```python
from build123d import *

# Parameters (mm, degrees)
ESTRUSIONE_SOTTILE1_DEPTH    = 6
RACCORDO3_R                  = 6
SCHIZZO4_R                   = 2
TAGLIO_ESTRUSIONE1_DEPTH     = 0.75
RACCORDO1_R                  = 0.75
RACCORDO2_R                  = 0.5
TAGLIO_ESTRUSIONE2_DEPTH     = 0.75
SCHIZZO6_R                   = 2
ESTRUSIONE_ESTRUSIONE1_DEPTH = 0.75
ESTRUSIONE_ESTRUSIONE3_DEPTH = 6
RACCORDO3_OF_SPECCHIA2_R     = 6
RACCORDO1_OF_SPECCHIA2_R     = 0.75
RACCORDO2_OF_SPECCHIA2_R     = 0.5
SCHIZZO8_R                   = 2
TAGLIO_ESTRUSIONE3_DEPTH     = 0.75
SCHIZZO9_R                   = 2
TAGLIO_ESTRUSIONE4_DEPTH     = 19


with BuildPart() as part:
    # Schizzo1 → Estrusione-Sottile1 (new, symmetric)
    with BuildSketch(Plane.XY):
        Polygon((0, 13), (0, 0), (-11, 0), (-11, 0.75), (-0.75, 0.75), (-0.75, 13), align=None)
    estrusione_sottile1 = extrude(amount=ESTRUSIONE_SOTTILE1_DEPTH, both=True)

    # Raccordo3
    raccordo3_edges = [part.edges().sort_by_distance(p)[0] for p in [
        (-11, 0.375, 6),
        (-11, 0.375, -6),
        (-0.375, 13, -6),
        (-0.375, 13, 6),
    ]]
    fillet(raccordo3_edges, radius=RACCORDO3_R - 0.0001)  # a hair under: the kernel refuses the full size

    # Schizzo4 → Taglio-Estrusione1 (cut)
    with BuildSketch(Plane(origin=(0, 0.75, 0), x_dir=(1, 0, 0), z_dir=(0, 1, 0))):
        with Locations(Location((-7, 0, 0), (0, 0, 180))):
            Circle(SCHIZZO4_R)
    taglio_estrusione1 = extrude(amount=-TAGLIO_ESTRUSIONE1_DEPTH, mode=Mode.SUBTRACT)

    # Raccordo1
    raccordo1_edges = [part.edges().sort_by_distance(p)[0] for p in [
        (0, 0, 0),
    ]]
    fillet(raccordo1_edges, radius=RACCORDO1_R)

    # Raccordo2
    raccordo2_edges = [part.edges().sort_by_distance(p)[0] for p in [
        (-0.75, 0.75, 0),
    ]]
    fillet(raccordo2_edges, radius=RACCORDO2_R)

    # Schizzo5 → Taglio-Estrusione2 (cut)
    with BuildSketch(Plane.ZY.offset(0.75)):
        with BuildLine():
            Line((2, 9), (2, 3.5))
            ThreePointArc((2, 3.5), (0, 1.5), (-2, 3.5))
            Line((-2, 3.5), (-2, 9))
            ThreePointArc((-2, 9), (0, 11), (2, 9))
        make_face()
    extrude(amount=-TAGLIO_ESTRUSIONE2_DEPTH, mode=Mode.SUBTRACT)

    # Schizzo6 → Estrusione-Estrusione1 (add)
    with BuildSketch(Plane(origin=(0, 0.75, 0), x_dir=(1, 0, 0), z_dir=(0, 1, 0))):
        with BuildLine():
            Line((-4.125, -6), (-7, -6))
            ThreePointArc((-7, -6), (-13, 0), (-7, 6))
            Line((-7, 6), (-4.125, 6))
            Line((-4.125, 6), (-4.125, -6))
        make_face()
        with Locations(Location((-7, 0, 0), (0, 0, 180))):
            Circle(SCHIZZO6_R, mode=Mode.SUBTRACT)
    estrusione_estrusione1 = extrude(amount=-ESTRUSIONE_ESTRUSIONE1_DEPTH)

    # Schizzo7 → Estrusione-Estrusione3 (add, symmetric)
    with BuildSketch(Plane.XY):
        with BuildLine():
            Line((-0.75, 13), (-0.75, 7))
            Line((-0.75, 7), (-0.75, 1.25))
            ThreePointArc((-0.75, 1.25), (-0.896446609, 0.896446609), (-1.25, 0.75))
            Line((-1.25, 0.75), (-4.125, 0.75))
            Line((-4.125, 0.75), (-4.125, 0))
            Line((-4.125, 0), (-0.75, 0))
            ThreePointArc((-0.75, 0), (-0.219669914, 0.219669914), (0, 0.75))
            Line((0, 0.75), (0, 7))
            Line((0, 7), (0, 13))
            Line((0, 13), (0, 13.5))
            ThreePointArc((0, 13.5), (0.073223305, 13.676776695), (0.25, 13.75))
            Line((0.25, 13.75), (5.5, 13.75))
            Line((5.5, 13.75), (5.5, 14.5))
            Line((5.5, 14.5), (0.25, 14.5))
            ThreePointArc((0.25, 14.5), (-0.457106781, 14.207106781), (-0.75, 13.5))
            Line((-0.75, 13.5), (-0.75, 13))
        make_face()
    estrusione_estrusione3 = extrude(amount=ESTRUSIONE_ESTRUSIONE3_DEPTH, both=True)


with BuildPart() as specchia2_1:
    # Specchia2: Estrusione-Sottile1 across plane
    add(estrusione_sottile1.mirror(Plane(origin=(5.5, 14.5, 6), x_dir=(0, 0, 1), z_dir=(-1, 0, 0))))

    # Specchia2 2: Taglio-Estrusione1 across plane
    add(taglio_estrusione1.mirror(Plane(origin=(5.5, 14.5, 6), x_dir=(0, 0, 1), z_dir=(-1, 0, 0))), mode=Mode.SUBTRACT)

    # Raccordo3 of Specchia2
    raccordo3_of_specchia2_edges = [specchia2_1.edges().sort_by_distance(p)[0] for p in [
        (22, 0.375, 6),
        (22, 0.375, -6),
        (11.375, 13, -6),
        (11.375, 13, 6),
    ]]
    fillet(raccordo3_of_specchia2_edges, radius=RACCORDO3_OF_SPECCHIA2_R - 0.0001)  # a hair under: the kernel refuses the full size

    # Raccordo1 of Specchia2
    raccordo1_of_specchia2_edges = [specchia2_1.edges().sort_by_distance(p)[0] for p in [
        (11, 0, 0),
    ]]
    fillet(raccordo1_of_specchia2_edges, radius=RACCORDO1_OF_SPECCHIA2_R)

    # Raccordo2 of Specchia2
    raccordo2_of_specchia2_edges = [specchia2_1.edges().sort_by_distance(p)[0] for p in [
        (11.75, 0.75, 0),
    ]]
    fillet(raccordo2_of_specchia2_edges, radius=RACCORDO2_OF_SPECCHIA2_R)


with BuildPart() as specchia2_3_1:
    # Specchia2 3: Estrusione-Estrusione1, Estrusione-Estrusione3 across plane
    add(estrusione_estrusione1.mirror(Plane(origin=(5.5, 14.5, 6), x_dir=(0, 0, 1), z_dir=(-1, 0, 0))))
    add(estrusione_estrusione3.mirror(Plane(origin=(5.5, 14.5, 6), x_dir=(0, 0, 1), z_dir=(-1, 0, 0))))


with BuildPart() as part_1:
    add(part.part)

    # Specchia2 united with what the copies to: union Specchia2_1, Specchia2 3_1
    add(specchia2_1.part)
    add(specchia2_3_1.part)

    # Schizzo8 → Taglio-Estrusione3 (cut)
    with BuildSketch(Plane(origin=(0, 14.5, 0), x_dir=(1, 0, 0), z_dir=(0, 1, 0))):
        with Locations(Location((5.5, 0, 0), (0, 0, 270))):
            Circle(SCHIZZO8_R)
    extrude(amount=-TAGLIO_ESTRUSIONE3_DEPTH, mode=Mode.SUBTRACT)

    # Schizzo9 → Taglio-Estrusione4 (cut)
    with BuildSketch(Plane(origin=(11.75, 0, 0), x_dir=(0, 0, -1), z_dir=(1, 0, 0))):
        with Locations((0, 7.375)):
            Circle(SCHIZZO9_R)
    extrude(amount=-TAGLIO_ESTRUSIONE4_DEPTH, mode=Mode.SUBTRACT)


solid = part_1.part
```
The model under review builds one solid part; all positions refer to its coordinate system, in mm. A direction names the side the tool comes from. Round coordinates to 2 decimals unless told otherwise and drop trailing zeros. Loops run counter-clockwise (first coordinate to the right, second up) from the corner with the lowest first, then second, coordinate; pieces in that order, holes last.
Item 1: Take a section at C-C (y = 5.75). Write out the cut boundary in (x, z), then the cut area to 3 significant figures.
Determined:
outline: (-0.75, -6) - (0, -6) - (0, -1.17) - (-0.75, -1.17) - close; (-0.75, 1.17) - (0, 1.17) - (0, 6) - (-0.75, 6) - close; (11, -6) - (11.75, -6) - (11.75, -1.17) - (11, -1.17) - close; (11, 1.17) - (11.75, 1.17) - (11.75, 6) - (11, 6) - close
area: 14.5 mm2
Item 2: For faces 4 (the face through (0, 7, 3)), 5 (the face through (11.38, 9.36, 0.26)), 6 (the face through (15.6, 0.75, 0.1)), 7 (the face through (-4.6, 0.75, 0.1)), list the 3-axis set-ups (+Z, -Z, +X, -X, +Y, -Y) from which the entire face can be reached by the end or side of a thin tool; tool diameter is ignored.
Determined:
face 4: +Z, -Z, -Y
face 5: +X, -X
face 6: +Z, -Z, +X, +Y
face 7: +Z, -Z, -X, +Y
Item 3: Mouldability with a two-part tool opening along X and no side actions: class faces 1 (the face through (-0.449, 14.215, 0.084)), 2 (the face through (-5, 0, 1)), 3 (the face through (-5.002, 0.38, 0.088)) as released by +X, released by -X, zero draft, split by the parting line, or undercut.
Determined:
face 1: released by -X
face 2: zero draft
face 3: undercut
Item 4: Take a section at D-D (z = 0). Give the number of separate pieces and of enclosed holes in the cut face, then the cut area to 3 significant figures.
Determined:
separate pieces: 6
enclosed holes: 0
area: 32.8 mm2
Item 5: For line 1 (X direction, y = 1.5, z = -4.5); line 2 (Y direction, x = -8, z = -2); line 3 (Y direction, x = 10.5, z = 5), list the stretches that pass through material, from the lowest coordinate up.
Determined:
line 1: x = -0.75 to 0, 11 to 11.75
line 2: y = 0 to 0.75
line 3: y = 13.75 to 14.5
Item 6: Take a section at B-B (y = 11.25). Write out the cut boundary in (x, z), then the cut area to 3 significant figures.
Determined:
outline: (-0.75, -6) - (0, -6) - (0, 6) - (-0.75, 6) - close; (11, -6) - (11.75, -6) - (11.75, 6) - (11, 6) - close
area: 18.0 mm2
Item 7: Take a section at A-A (x = 5.5). Write out the cut boundary in (y, z).
Determined:
outline: (13.75, -6) - (14.5, -6) - (14.5, -2) - (13.75, -2) - close; (13.75, 2) - (14.5, 2) - (14.5, 6) - (13.75, 6) - close
Item 8: Clearance check with flat-ended pins moving along their axes: pin 1 Ø6 at (y, z) = (5.5, 4) entering from +X; pin 2 Ø4.5 at (x, z) = (18, 0) entering from -Y; pin 3 Ø4 at (y, z) = (5, 4.5) entering from -X; pin 4 Ø3.5 at (x, z) = (16, -0.5) entering from +Y. State where each tip first meets the part, or that it passes through.
Determined:
pin 1: stops at x = 11.75
pin 2: stops at y = 0
pin 3: stops at x = -0.75
pin 4: stops at y = 0.75
